Build history of the part. All positions in model axes, mm. Give positions to 0.01 mm unless a question says otherwise; leave off trailing zeros. Write each loop counter-clockwise with the first axis right and the second up, starting at its lowest first coordinate (ties: lowest second). Pieces come first, ordered by that corner, then holes. Notation, with made-up numbers: (-33, -17.5) -> (-14, -17.5) arc R11 ccw to (-14, -0.5) -> close; hole circle Ø11 at (-26.75, -11). An arc over 180 degrees is marked (long way). One line per question, with ' | ' between items. Start each with the question number.
(1) Band-saw the part on C-C, the plane x = 4.5. Give the cut face in (y, z), and give its area (3 significant figures).
(2) Band-saw the part on A-A, the plane x = 0. Give the cut face in (y, z).
(3) Band-saw the part on D-D, the plane y = -21.25. Give the cut face in (x, z), and give its area (3 significant figures).
(4) Pull direction Y, two halves, no side cores. Call faces 1 (the cylindrical face through (0.99, -0.76, -0.03)), 2 (the flat face through (9, -7, 0)), 3 (the flat face through (-6, -21, 0)): released by +Y, released by -Y, zero draft, split by the parting line, or undercut.
(5) Band-saw the part on B-B, the plane z = 0.95. Give the cut face in (x, y) (3 decimals), and give its area (3 significant figures).
(6) Pin check, flat tip, straight feed: P1, Ø2.5, axis at x = 0, y = -9.268, coming from the +Z side. Stop position of the tip, or through.
(7) Drill centre lines: probe 1 along X at (y, z) = (0, -0.25) (3 decimals); probe 2 along Y at (x, z) = (0, 0.2); probe 3 along Y at (x, z) = (-1, -0.75). Where is each one in solid material? Low to high. Write a range as from..to.
from build123d import *

# Parameters (mm, degrees)
SKETCH1_W            = 18
SKETCH1_H            = 10
BOSS_EXTRUDE1_DEPTH  = 2
SKETCH2_W            = 18
SKETCH2_H            = 19
BOSS_EXTRUDE2_DEPTH  = 2
M3_CLEARANCE_HOLE1_D = 3.2
CHAMFER1_SIZE        = 6
M3_TAPPED_HOLE1_D    = 2.5


with BuildPart() as part:
    # Sketch1 → Boss-Extrude1 (new, symmetric)
    with BuildSketch(Plane.XY):
        Rectangle(SKETCH1_W, SKETCH1_H)
    extrude(amount=BOSS_EXTRUDE1_DEPTH, both=True)

    # Sketch2 → Boss-Extrude2 (add, symmetric)
    with BuildSketch(Plane.XY):
        with Locations((0, -14.5)):
            Rectangle(SKETCH2_W, SKETCH2_H)
    extrude(amount=BOSS_EXTRUDE2_DEPTH, both=True)

    # M3 Clearance Hole1 (through all)
    with Locations(Plane(origin=(0, 0, 2), x_dir=(-1, 0, 0), z_dir=(0, 0, 1))):
        with Locations((0, 9.268), (0, 20.698), (-5.715, -0.0028), (5.715, -0.0028)):
            Hole(M3_CLEARANCE_HOLE1_D / 2)

    # Chamfer1
    chamfer1_edges = [part.edges().sort_by_distance(p)[0] for p in [
        (-9, -24, 0),
        (9, -24, 0),
    ]]
    chamfer(chamfer1_edges, length=CHAMFER1_SIZE)

    # M3 Tapped Hole1 (through all)
    with Locations(Plane.XY.offset(2)):
        with Locations((0, -14.983), (0, 0.0028)):
            Hole(M3_TAPPED_HOLE1_D / 2)


solid = part.part
Results:
1) outline: (-22.5, -2) -> (-1.04, -2) -> (-1.04, 2) -> (-22.5, 2) -> close; (1.04, -2) -> (5, -2) -> (5, 2) -> (1.04, 2) -> close | area: 102 mm²
2) outline: (-24, -2) -> (-22.3, -2) -> (-22.3, 2) -> (-24, 2) -> close; (-19.1, -2) -> (-16.23, -2) -> (-16.23, 2) -> (-19.1, 2) -> close; (-13.73, -2) -> (-10.87, -2) -> (-10.87, 2) -> (-13.73, 2) -> close; (-7.67, -2) -> (-1.25, -2) -> (-1.25, 2) -> (-7.67, 2) -> close; (1.25, -2) -> (5, -2) -> (5, 2) -> (1.25, 2) -> close
3) outline: (-5.75, -2) -> (-1.5, -2) -> (-1.5, 2) -> (-5.75, 2) -> close; (1.5, -2) -> (5.75, -2) -> (5.75, 2) -> (1.5, 2) -> close | area: 34.0 mm²
4) face 1: undercut | face 2: zero draft | face 3: released by -Y
5) outline: (-9, -18) -> (-3, -24) -> (3, -24) -> (9, -18) -> (9, 5) -> (-9, 5) -> close; hole circle Ø3.2 at (-5.715, 0.003); hole circle Ø3.2 at (0, -20.698); hole circle Ø3.2 at (0, -9.268); hole circle Ø2.5 at (0, -14.983); hole circle Ø2.5 at (0, 0.003); hole circle Ø3.2 at (5.715, 0.003) | area: 444 mm²
6) P1: passes through
7) probe 1: x = -9..-7.315, -4.115..-1.25, 1.25..4.115, 7.315..9 | probe 2: y = -24..-22.3, -19.1..-16.23, -13.73..-10.87, -7.67..-1.25, 1.25..5 | probe 3: y = -24..-21.95, -19.45..-15.73, -14.23..-10.52, -8.02..-0.75, 0.75..5
